Work out the finished part from the listing and answer in its coordinate system (mm). Face numbers are marked on the shaded views. A direction names the side the tool comes from. Give positions to 0.01 mm unless a question says otherwise; leave off trailing zeros. Loops run counter-clockwise (first coordinate to the right, second up) from the corner with the lowest first, then second, coordinate; pieces in that order, holes last. Notation, with made-up numbers: (19.5, -36) - (67.5, -36) arc R22 ccw to (67.5, -26) - close; hole circle Ø9 at (65, -22). An arc over 180 degrees is marked (long way). One line per question, with ' | ' between items.
from build123d import *

# Parameters (mm, degrees)
F0_R      = 2.921
F3_R      = 2.921
F4_FACE_R = 2.921
F8_R      = 2.54
F9_DEPTH  = 6.096


with BuildPart() as f4:
    # F0 (on Top) → F4 section 0
    with BuildSketch(Plane.XY):
        with Locations((9.144, 0)):
            Circle(F0_R)
    # F3 (on offset) → F4 section 1
    with BuildSketch(Plane.XY.offset(6.096)):
        with Locations((9.144, 0)):
            Circle(F3_R)
    loft()

    # F6: sweep along a path in F5
    with BuildLine(Plane.XZ) as f6_path:
        ThreePointArc((9.144, 6.096), (0, 15.24), (-9.144, 6.096))
    # F4_face (on face) → F6 (sweep)
    with BuildSketch(Plane(origin=(9.144, 0, 6.096), x_dir=(1, 0, 0), z_dir=(0, 0, 1))):
        Circle(F4_FACE_R)
    sweep(path=f6_path.line)

    # F7: F4 across plane


with BuildPart() as f4_1:
    add(f4.part)
    add(f4.part.mirror(Plane.YZ))

    # F8 (on Top) → F9 (join)
    with BuildSketch(Plane.XY):
        with BuildLine():
            Line((7.9841911765, -2.6808738301), (15.2586764706, -5.8279865872))
            ThreePointArc((15.2586764706, -5.8279865872), (24.13, 0), (15.2586764706, 5.8279865872))
            Line((15.2586764706, 5.8279865872), (7.9841911765, 2.6808738301))
            ThreePointArc((7.9841911765, 2.6808738301), (6.223, 0), (7.9841911765, -2.6808738301))
        make_face()
        with Locations((17.78, 0)):
            Circle(F8_R, mode=Mode.SUBTRACT)
    extrude(amount=F9_DEPTH)

    # F10: F4 across plane


with BuildPart() as f4_2:
    add(f4_1.part)
    add(f4_1.part.mirror(Plane.YZ))


solid = f4_2.part
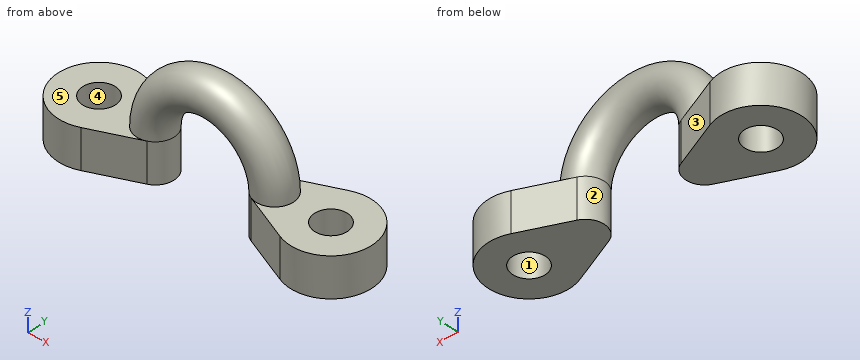
1. Determine the mould class of the marked faces 3, 4 and 5 for opening direction Y: +Y half, -Y half, draft (parallel to the pull), parting line (faces both ways), or undercut.
Evaluation:
face 3: +Y half | face 4: undercut | face 5: draft
2. Find section D-D on y = 4.25. Write down the section's boundary in (x, z).
Evaluation:
outline: (-22.5, 0) - (-11.61, 0) - (-11.61, 6.1) - (-22.5, 6.1) - close; (11.61, 0) - (22.5, 0) - (22.5, 6.1) - (11.61, 6.1) - close
3. Flat-ended cylindrical pins translate along their axes: pin 1 (5 mm diameter, centred on y = -1, z = 13.5, fed in from +X); pin 2 (6 mm diameter, centred on x = 17.78, y = 0, fed in from +Z); pin 3 (4 mm diameter, centred on x = -8, z = 14, fed in from +Y). Find the tip coordinate at first contact, or state that the pin passes through.
Evaluation:
pin 1: x = 10.96 | pin 2: z = 6.1 | pin 3: y = 2.92
4. Find section C-C on y = 0. Write down the section's boundary in (x, z) (3 decimals).
Evaluation:
outline: (-24.13, 0) - (-20.32, 0) - (-20.32, 6.096) - (-24.13, 6.096) - close; (-15.24, 0) - (-6.223, 0) - (-6.223, 6.096) arc R6.223 cw to (6.223, 6.096) - (6.223, 0) - (15.24, 0) - (15.24, 6.096) - (12.065, 6.096) arc R12.065 ccw to (-12.065, 6.096) - (-15.24, 6.096) - close; (20.32, 0) - (24.13, 0) - (24.13, 6.096) - (20.32, 6.096) - close
5. Which of the six approach directions +Z, -Z, +X, -X, +Y, -Y give full straight-line access (tool end or side, diameter ignored) to the marked faces 1 and 2?
Evaluation:
face 1: +Z, -Z | face 2: -Z
6. Find section B-B on x = -17.78. Write down the section's boundary in (y, z), then the cut area to 3 significant figures.
Evaluation:
outline: (-6.35, 0) - (-2.54, 0) - (-2.54, 6.1) - (-6.35, 6.1) - close; (2.54, 0) - (6.35, 0) - (6.35, 6.1) - (2.54, 6.1) - close | area: 46.5 mm2
7. Consider L1, parallel to Y at x = 17.78, z = 3.25; L2, parallel to Z at x = -20, y = 1.5; L3, parallel to Y at x = -18.5, z = 3. Determine where each line is inside the solid, lowest interval first.
Evaluation:
L1: -6.35 to -2.54, 2.54 to 6.35 | L2: 0 to 6.1 | L3: -6.31 to -2.44, 2.44 to 6.31
8. Find section A-A on z = 4.25. Write down the section's boundary in (x, y), then the cut area to 3 significant figures.
Evaluation:
outline: (-15.26, -5.83) - (-7.98, -2.68) arc R2.92 ccw to (-7.98, 2.68) - (-15.26, 5.83) arc R6.35 ccw (long way) to start; (7.98, -2.68) - (15.26, -5.83) arc R6.35 ccw (long way) to (15.26, 5.83) - (7.98, 2.68) arc R2.92 ccw to start; hole circle Ø5.08 at (-17.78, 0); hole circle Ø5.08 at (17.78, 0) | area: 286 mm2
